Autodesk Inventor part; units mm, degrees
ref_plane "YZ Plane" through (0, 0, 0) normal (1, 0, 0) x (0, 1, 0)
ref_plane "XZ Plane" through (0, 0, 0) normal (0, 1, 0) x (-1, 0, 0)
ref_plane "XY Plane" through (0, 0, 0) normal (0, 0, 1) x (1, 0, 0)
sketch "Sketch1" plane through (0, 0, 0) normal (0, 0, 1) x (1, 0, 0)
  line L0 (-30.7315, 6.2426) -> (-22.7315, 6.2426)
  line L1 (-22.7315, 6.2426) -> (-22.7315, -8.7574)
  line L2 (-22.7315, -8.7574) -> (-30.7315, -8.7574)
  line L3 (-30.7315, -8.7574) -> (-30.7315, 6.2426)
  line L4 (-6.7315, 2.2426) -> (-6.7315, 21.2426)
  line L5 (-6.7315, 21.2426) -> (-22.7315, 21.2426)
  line L6 (-22.7315, 21.2426) -> (-22.7315, 6.2426)
  line L7 (-22.7315, -8.7574) -> (-6.7315, 2.2426)
  point P0 (0, 0)
  dimension "d0" = 15
  dimension "d1" = 8
  dimension "d2" = 15
  dimension "d3" = 16
  dimension "d4" = 19
extrude "Extrusion1" add sketch "Sketch1" along normal blind 16
sketch "Sketch2" plane through (-22.7315, 21.2426, 0) normal (0, 1, 0) x (1, 0, 0)
  line L0 (16, 0) -> (16, -16)
  line L1 (0, -5.3333) -> (16, -5.3333)
  line L2 (16, -5.3333) -> (16, -10.6667)
  line L3 (16, -10.6667) -> (0, -10.6667)
  line L4 (0, -10.6667) -> (0, -5.3333)
  line L5 (0, 0) -> (0, -16)
  line L6 (16, 0) -> (0, 0)
  line L7 (16, -16) -> (0, -16)
  point P0 (22.7315, 0)
  dimension "d7" = 16
  dimension "d8" = 5.3333
  dimension "d9" = 5.3333
extrude "Extrusion2" cut sketch "Sketch2" against normal blind 2 contours L0 L3 L4 L1
sketch "Sketch3" plane through (-6.7315, 2.2426, 0) normal (1, 0, 0) x (0, 0, -1)
  line L0 (-10.6667, 17) -> (-10.6667, 19)
  line L1 (-10.6667, 19) -> (-16, 19)
  line L2 (-16, 0) -> (-16, 19)
  line L3 (0, 0) -> (-16, 0)
  line L4 (0, 0) -> (0, 19)
  line L5 (0, 19) -> (-5.3333, 19)
  line L6 (-5.3333, 19) -> (-5.3333, 17)
  line L7 (-5.3333, 17) -> (-10.6667, 17)
  line L8 (0, 0) -> (-16, 0)
  line L9 (-10.6667, 17) -> (-5.3333, 17)
  line L10 (-10.6667, 17) -> (-10.6667, -2)
  line L11 (-10.6667, -2) -> (-5.3333, -2)
  line L12 (-5.3333, -2) -> (-5.3333, 17)
  point P0 (0, -2.2426)
  dimension "d14" = 19
  dimension "d15" = 19
extrude "Extrusion3" cut sketch "Sketch3" against normal blind 2 contours L7 L12 L3 L10 | L3 L12 L11 L10
sketch "Sketch4" plane through (-22.7315, -8.7574, 0) normal (0.5665, -0.824, 0) x (0.824, 0.5665, 0)
  line L0 (16.9894, 10.6667) -> (19.4165, 10.6667)
  line L1 (19.4165, 10.6667) -> (19.4165, 16)
  line L2 (0, 16) -> (19.4165, 16)
  line L3 (0, 0) -> (0, 16)
  line L4 (0, 0) -> (19.4165, 0)
  line L5 (19.4165, 0) -> (19.4165, 5.3333)
  line L6 (19.4165, 5.3333) -> (16.9894, 5.3333)
  line L7 (16.9894, 5.3333) -> (16.9894, 10.6667)
  line L8 (16.9894, 10.6667) -> (19.4165, 10.6667)
  line L9 (16.9894, 10.6667) -> (0, 10.6667)
  line L10 (0, 10.6667) -> (0, 5.3333)
  line L11 (0, 5.3333) -> (16.9894, 5.3333)
  line L12 (16.9894, 5.3333) -> (16.9894, 10.6667)
  point P0 (23.693, 0)
  dimension "d17" = 19.4165
extrude "Extrusion4" cut sketch "Sketch4" against normal blind 2 contours L7 L11 L3 L9
chamfer "Chamfer1" distance 2 angle 45 1 edges at (-23.8645, -7.1093, 8)
sketch "Sketch5" plane through (-30.7315, -8.7574, 0) normal (-1, 0, 0) x (0, 0, 1)
  line L0 (6, 13) -> (10, 13)
  line L1 (10, 13) -> (10, 2)
  line L2 (10, 2) -> (6, 2)
  line L3 (6, 2) -> (6, 13)
  line L4 (0, 15) -> (0, 0)
  line L5 (0, 0) -> (16, 0)
  line L6 (16, 15) -> (16, 0)
  line L7 (0, 15) -> (16, 15)
  point P0 (0, 8.7574)
  dimension "d23" = 4
  dimension "d24" = 11
  dimension "d25" = 6
  dimension "d26" = 15
  dimension "d27" = 16
  dimension "d28" = 2
extrude "Extrusion5" cut sketch "Sketch5" against normal blind 5 contours L0 L1 L2 L3
sketch "Sketch6" plane through (0, 0, 0) normal (0, 0, -1) x (-1, 0, 0)
  line L0 (6.7315, 2.2426) -> (6.7315, 21.2426)
  line L1 (22.7315, -8.7574) -> (6.7315, 2.2426)
  line L2 (30.7315, -8.7574) -> (22.7315, -8.7574)
  line L3 (30.7315, 6.2426) -> (30.7315, -8.7574)
  line L4 (22.7315, 6.2426) -> (30.7315, 6.2426)
  line L5 (22.7315, 21.2426) -> (22.7315, 6.2426)
  line L6 (6.7315, 21.2426) -> (22.7315, 21.2426)
  line L7 (20.9315, 19.4426) -> (20.9315, 4.4426)
  line L8 (20.9315, 4.4426) -> (28.9315, 4.4426)
  line L9 (28.9315, 4.4426) -> (28.9315, -6.9574)
  line L10 (28.9315, -6.9574) -> (23.2905, -6.9574)
  line L11 (23.2905, -6.9574) -> (8.5315, 3.1895)
  line L12 (8.5315, 3.1895) -> (8.5315, 19.4426)
  line L13 (8.5315, 19.4426) -> (20.9315, 19.4426)
  point P0 (0, 0)
  dimension "d31" = 1.8
extrude "Extrusion6" cut sketch "Sketch6" against normal blind 0.5 contours L7 L8 L9 L10 L11 L12 L13
sketch "Sketch7" plane through (0, 0, 16) normal (0, 0, 1) x (1, 0, 0)
  line L0 (-6.7315, 21.2426) -> (-22.7315, 21.2426)
  line L1 (-6.7315, 2.2426) -> (-6.7315, 21.2426)
  line L2 (-6.7315, 2.2426) -> (-6.7315, 21.2426)
  line L3 (-6.7315, 21.2426) -> (-22.7315, 21.2426)
  line L4 (-22.7315, 21.2426) -> (-22.7315, 6.2426)
  line L5 (-22.7315, 6.2426) -> (-30.7315, 6.2426)
  line L6 (-30.7315, 6.2426) -> (-30.7315, -8.7574)
  line L7 (-30.7315, -8.7574) -> (-22.7315, -8.7574)
  line L8 (-22.7315, -8.7574) -> (-6.7315, 2.2426)
  line L9 (-20.9315, 4.4426) -> (-20.9315, 19.4426)
  line L10 (-20.9315, 19.4426) -> (-8.5315, 19.4426)
  line L11 (-8.5315, 19.4426) -> (-8.5315, 3.1895)
  line L12 (-8.5315, 3.1895) -> (-23.2905, -6.9574)
  line L13 (-23.2905, -6.9574) -> (-28.9315, -6.9574)
  line L14 (-28.9315, -6.9574) -> (-28.9315, 4.4426)
  line L15 (-28.9315, 4.4426) -> (-20.9315, 4.4426)
  line L16 (-20.9315, 19.4426) -> (-20.9315, 4.4426)
  point P0 (0, 0)
  dimension "d34" = 0
extrude "Extrusion7" cut sketch "Sketch7" against normal blind 0.5 contours L9 L10 L11 L12 L13 L14 L15
equation "\"d8\" = 0.333333 * d7"
equation "\"d9\" = -2 * d8 + d7"
equation "\"d14\" = d15"
equation "\"d25\" = -0.5 * d23 + 0.5 * d27"
equation "\"d28\" = -0.5 * d24 + 0.5 * d26"
properties part number "under walle L3"
Here's how the part is built. I have some questions about the finished solid (model axes, mm). A direction names the side the tool comes from. Round coordinates to 2 decimals unless told otherwise and drop trailing zeros. Write each loop counter-clockwise with the first axis right and the second up, starting at its lowest first coordinate (ties: lowest second). Pieces come first, ordered by that corner, then holes.
Q1. If we mould it in two halves opening along Y, with no side actions, what happens to faces 5 (the flat face through (-16.01, -1.95, 0.25)), 6 (the flat face through (-28, -6.757, 8)), 7 (the flat face through (-16, 19.243, 8)), 8 (the flat face through (-22.732, 14, 8))? For each: +Y half, -Y half, draft (parallel to the pull), parting line (faces both ways), or undercut.
Q2. If we section it at A-A on x = -27: Write out the boundary of the cut face in (y, z), plus the area to 3 significant figures.
Q3. Which directions (+Z, -Z, +X, -X, +Y, -Y) give clear straight access to the entire face, cutting with the end or side of a thin tool? Please do faces 1 (the flat face through (-8.732, 10, 8)), 2 (the flat face through (-22.472, -7.346, 7.963)), 3 (the flat face through (-9.29, 1.68, 7.96)), 4 (the flat face through (-8, 16, 10.667)).
Q4. If we section it at C-C on y = 15.5: Write out the boundary of the cut face in (x, z), plus the area to 3 significant figures.
Q5. If we section it at D-D on x = -11.75: Write out the boundary of the cut face in (y, z), plus the area to 3 significant figures.
Q6. Please list where these lines run through material, in increasing order: probe 1 along Z at (x, y) = (-8.25, 18.5); probe 2 along Z at (x, y) = (-20, 3.5); probe 3 along X at (y, z) = (19, 6.75).
Q7. Will these pins go through, and if not, where does the flat tip stop? P1, Ø2.5, axis at x = -28.5, z = 10, coming from the +Y side; P2, Ø0.6, axis at y = 9, z = 0, coming from the -X side; P3, Ø1, axis at x = -10, y = 13.5, coming from the -Z side.
Answer below:
1. face 5: undercut
1. face 6: undercut
1. face 7: +Y half
1. face 8: draft
2. outline: (-8.76, 0) - (-6.96, 0) - (-6.96, 0.5) - (4.44, 0.5) - (4.44, 0) - (6.24, 0) - (6.24, 16) - (4.44, 16) - (4.44, 15.5) - (-6.96, 15.5) - (-6.96, 16) - (-8.76, 16) - close; hole (-6.76, 6) - (4.24, 6) - (4.24, 10) - (-6.76, 10) - close
2. area: 185 mm2
3. face 1: +X, +Y, -Y
3. face 2: +X, -Y
3. face 3: -Y
3. face 4: +X, +Y
4. outline: (-22.73, 0) - (-20.93, 0) - (-20.93, 0.5) - (-8.53, 0.5) - (-8.53, 0) - (-6.73, 0) - (-6.73, 5.33) - (-8.73, 5.33) - (-8.73, 10.67) - (-6.73, 10.67) - (-6.73, 16) - (-8.53, 16) - (-8.53, 15.5) - (-20.93, 15.5) - (-20.93, 16) - (-22.73, 16) - close
4. area: 233 mm2
5. outline: (-1.21, 0) - (0.98, 0) - (0.98, 0.5) - (19.44, 0.5) - (19.44, 0) - (21.24, 0) - (21.24, 5.33) - (19.24, 5.33) - (19.24, 10.67) - (21.24, 10.67) - (21.24, 16) - (19.44, 16) - (19.44, 15.5) - (0.98, 15.5) - (0.98, 16) - (-1.21, 16) - (-1.21, 10.67) - (1.22, 10.67) - (1.22, 5.33) - (-1.21, 5.33) - close
5. area: 317 mm2
6. probe 1: z = 0 to 5.33, 10.67 to 16
6. probe 2: z = 0.5 to 15.5
6. probe 3: x = -22.73 to -8.73
7. P1: stops at y = 6.24
7. P2: stops at x = -22.73
7. P3: stops at z = 0.5
